```python
from build123d import *

# Parameters (mm, degrees)
SALIENTE_EXTRUIR1_DEPTH = 760
CROQUIS3_W              = 441.770557025
CROQUIS3_H              = 21.549783269
CROQUIS3_H_2            = 18.85606036
CORTAR_EXTRUIR1_DEPTH   = 899


with BuildPart() as part:
    # Croquis2 → Saliente-Extruir1 (new body)
    with BuildSketch(Plane.XY):
        Polygon((0, 0), (0, 760), (1800, 760), (1800, 0), (1300, 0), (1300, 525.845869983), (1750.467945366, 525.845869983), (1750.467945366, 724.319370664), (47.213684499, 724.319370664), (47.213684499, 0), align=None)
    extrude(amount=SALIENTE_EXTRUIR1_DEPTH)

    # Croquis3 → Cortar-Extruir1 (cut)
    with BuildSketch(Plane.XY.offset(760)):
        with Locations((1553.640740137, 357.52664055)):
            Rectangle(CROQUIS3_W, CROQUIS3_H)
        with Locations((1553.640740137, 162.23172967)):
            Rectangle(CROQUIS3_W, CROQUIS3_H_2)
    extrude(amount=-CORTAR_EXTRUIR1_DEPTH, mode=Mode.SUBTRACT)


solid = part.part
```
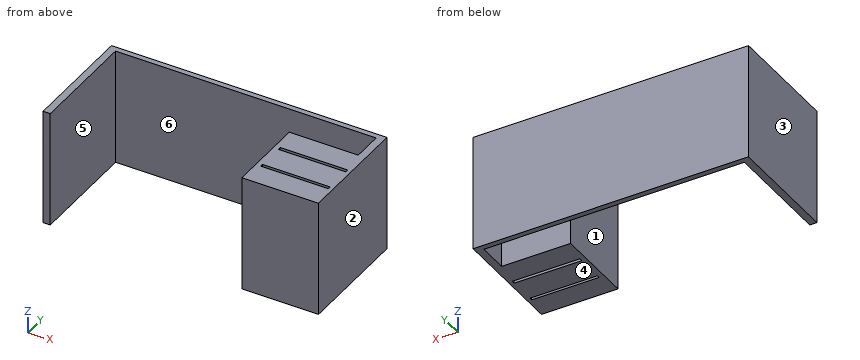
The model under review builds one solid part; all positions refer to its coordinate system, in mm. Face numbers are marked on the shaded views. A direction names the side the tool comes from. Round coordinates to 2 decimals unless told otherwise and drop trailing zeros. Order: outer loops, then holes, each group sorted by start corner. A loop starts at its lowest first (then second) coordinate and runs counter-clockwise, first axis right, second up. Notation, with made-up numbers: (0.5, -10.75) -> (13.5, -10.75) arc R16 ccw to (13.5, 12.25) -> close; hole circle Ø10 at (83, -35.5). An arc over 180 degrees is marked (long way). Use a Markdown table: item, result.
Q1. For line 1 (X direction, y = 166, z = 257); line 2 (Y direction, x = 1617.5, z = 457); line 3 (X direction, y = 682.5, z = 180), list the stretches that pass through material, from the lowest coordinate up.
Values:
| item | result |
|---|---|
| line 1 | x = 0 to 47.21, 1300 to 1332.76, 1774.53 to 1800 |
| line 2 | y = 0 to 152.8, 171.66 to 346.75, 368.3 to 525.85, 724.32 to 760 |
| line 3 | x = 0 to 47.21, 1750.47 to 1800 |
Q2. Mouldability with a two-part tool opening along X and no side actions: class the marked faces 1, 2 and 3 as +X half, -X half, draft (parallel to the pull), parting line (faces both ways), or undercut.
Values:
| item | result |
|---|---|
| face 1 | undercut |
| face 2 | +X half |
| face 3 | -X half |
Q3. We need section C-C on z = 463. Write out the cut boundary in (x, y).
Values:
| item | result |
|---|---|
| outline | (0, 0) -> (47.21, 0) -> (47.21, 724.32) -> (1750.47, 724.32) -> (1750.47, 525.85) -> (1300, 525.85) -> (1300, 0) -> (1800, 0) -> (1800, 760) -> (0, 760) -> close; hole (1332.76, 152.8) -> (1774.53, 152.8) -> (1774.53, 171.66) -> (1332.76, 171.66) -> close; hole (1332.76, 346.75) -> (1774.53, 346.75) -> (1774.53, 368.3) -> (1332.76, 368.3) -> close |
Q4. We need section B-B on x = 1413. Write out the cut boundary in (y, z), then the cut area to 3 significant figures.
Values:
| item | result |
|---|---|
| outline | (0, 0) -> (152.8, 0) -> (152.8, 760) -> (0, 760) -> close; (171.66, 0) -> (346.75, 0) -> (346.75, 760) -> (171.66, 760) -> close; (368.3, 0) -> (525.85, 0) -> (525.85, 760) -> (368.3, 760) -> close; (724.32, 0) -> (760, 0) -> (760, 760) -> (724.32, 760) -> close |
| area | 396,000 mm^2 |
Q5. We need section A-A on y = 428.5. Write out the cut boundary in (x, z).
Values:
| item | result |
|---|---|
| outline | (0, 0) -> (47.21, 0) -> (47.21, 760) -> (0, 760) -> close; (1300, 0) -> (1800, 0) -> (1800, 760) -> (1300, 760) -> close |
Q6. Clearance check with a flat-ended pin moving along its axis: P1, Ø3, axis at x = 388.5, z = 270, coming from the -Y side. State where the tip first meets the part, or that it passes through.
Values:
| item | result |
|---|---|
| P1 | stops at y = 724.32 |
Q7. Tool access review of the marked faces 4, 5 and 6: name each direction out of +Z, -Z, +X, -X, +Y, -Y from which nothing blocks a thin tool from reaching the whole face with its end or side.
Values:
| item | result |
|---|---|
| face 4 | -Z, +X, -X, +Y, -Y |
| face 5 | +Z, -Z, -Y |
| face 6 | +Z, -Z |
Q8. We need section D-D on y = 699. Write out the cut boundary in (x, z).
Values:
| item | result |
|---|---|
| outline | (0, 0) -> (47.21, 0) -> (47.21, 760) -> (0, 760) -> close; (1750.47, 0) -> (1800, 0) -> (1800, 760) -> (1750.47, 760) -> close |
